Geometry check sheet. Reference: the model listing, model coordinates, mm. A direction names the side the tool comes from. Coordinates: 2 decimals unless noted, no trailing zeros. Loops run counter-clockwise (first coordinate to the right, second up) from the corner with the lowest first, then second, coordinate; pieces in that order, holes last.
from build123d import *

# Parameters (mm, degrees)
SKETCH_R     = 1.6
PAD_DEPTH    = 4
CHAMFER_SIZE = 0.5
POCKET_DEPTH = 10.001


with BuildPart() as part:
    # Sketch → Pad (new body)
    with BuildSketch(Plane.XY):
        with BuildLine():
            ThreePointArc((-15, 5), (-20, 0), (-15, -5))
            Line((-15, -5), (15, -5))
            ThreePointArc((15, -5), (20, 0), (15, 5))
            Line((-15, 5), (15, 5))
        make_face()
        with Locations((-15, 0)):
            Circle(SKETCH_R, mode=Mode.SUBTRACT)
        with Locations((15, 0)):
            Circle(SKETCH_R, mode=Mode.SUBTRACT)
    extrude(amount=PAD_DEPTH)

    # Chamfer
    chamfer_edges = [part.edges().sort_by_distance(p)[0] for p in [
        (-20, 0, 4),
        (0, -5, 4),
        (20, 0, 4),
        (0, 5, 4),
        (13.4, 0, 4),
        (-16.6, 0, 4),
        (-20, 0, 0),
        (0, -5, 0),
        (20, 0, 0),
        (0, 5, 0),
        (13.4, 0, 0),
        (-16.6, 0, 0),
    ]]
    chamfer(chamfer_edges, length=CHAMFER_SIZE)

    # Sketch001 → Pocket (cut, through all)
    with BuildSketch(Plane.XZ.offset(5)):
        Polygon((-12.5, 4.5), (-10.5, 2), (10.5, 2), (12.5, 4.5), align=None)
    extrude(amount=-POCKET_DEPTH, mode=Mode.SUBTRACT)


solid = part.part
(1) Sectioned sample at A-A on z = 2.5. Record the cut outline in (x, y), and give its area (3 significant figures).
Findings:
outline: (-15, -5) - (-10.9, -5) - (-10.9, 5) - (-15, 5) arc R5 ccw to start; (10.9, -5) - (15, -5) arc R5 ccw to (15, 5) - (10.9, 5) - close; hole circle Ø3.2 at (-15, 0); hole circle Ø3.2 at (15, 0)
area: 144 mm2
(2) Sectioned sample at C-C on x = -5. Record the cut outline in (y, z).
Findings:
outline: (-5, 0.5) - (-4.5, 0) - (4.5, 0) - (5, 0.5) - (5, 2) - (-5, 2) - close
(3) Sectioned sample at B-B on y = 0. Record the cut outline in (x, z), and give its area (3 significant figures).
Findings:
outline: (-20, 0.5) - (-19.5, 0) - (-17.1, 0) - (-16.6, 0.5) - (-16.6, 3.5) - (-17.1, 4) - (-19.5, 4) - (-20, 3.5) - close; (-13.4, 0.5) - (-12.9, 0) - (12.9, 0) - (13.4, 0.5) - (13.4, 3.5) - (12.9, 4) - (12.1, 4) - (10.5, 2) - (-10.5, 2) - (-12.1, 4) - (-12.9, 4) - (-13.4, 3.5) - close; (16.6, 0.5) - (17.1, 0) - (19.5, 0) - (20, 0.5) - (20, 3.5) - (19.5, 4) - (17.1, 4) - (16.6, 3.5) - close
area: 87.7 mm2
(4) Draft check along Y on faces 3 (the cylindrical face through (20, 0, 2)), 4 (the flat face through (-0.2, -5, 1.6)), 5 (the flat face through (11.3, -0.1, 3)), 6 (the cylindrical face through (-16.6, 0.07, 1.98)). Enter one of: +Y half, -Y half, draft (parallel to the pull), parting line (faces both ways), or undercut.
Findings:
face 3: parting line
face 4: -Y half
face 5: draft
face 6: undercut
(5) Scan lines: L1, parallel to Y at x = 15, z = 2.75; L2, parallel to X at y = -0.75, z = 2.15; L3, parallel to Z at x = 1, y = -3.25. Record each from-to range of solid material in increasing order.
Findings:
L1: y = -5 to -1.6, 1.6 to 5
L2: x = -19.94 to -16.41, -13.59 to -10.62, 10.62 to 13.59, 16.41 to 19.94
L3: z = 0 to 2
(6) Gauge pin test, flat ends, axial feed: pin 1 Ø1 at (y, z) = (2.5, 1.5) entering from +X; pin 2 Ø3 at (x, y) = (-9.5, 3) entering from +Z (3 decimals); pin 3 Ø3 at (x, y) = (15, 0) entering from -Z; pin 4 Ø6 at (x, y) = (0.5, -2) entering from +Z. Record the tip position at first contact, or that the pin passes through.
Findings:
pin 1: stops at x = 19.58
pin 2: stops at z = 2.625
pin 3: passes through
pin 4: stops at z = 2
(7) Access from +Z, -Z, +X, -X, +Y, -Y to the whole of each face (thin tool, end or side, straight path). Record for faces 1 (the flat face through (-11.3, -0.1, 3)), 2 (the cylindrical face through (-20, 0, 2)).
Findings:
face 1: +Z, +Y, -Y
face 2: +Z, -Z, -X
